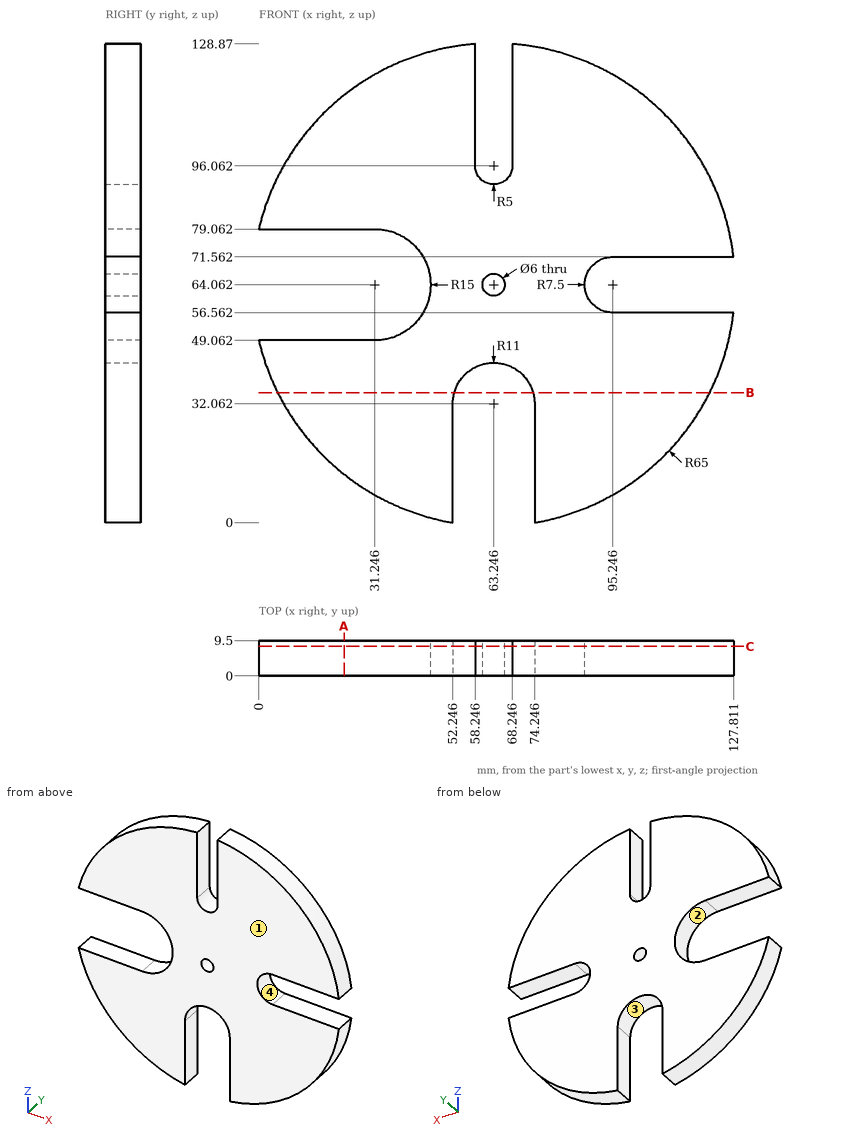
Could you check a few things on this drawing? It's one solid part, dimensions in mm from its lowest x, y, z. Coordinates: 2 decimals unless noted, no trailing zeros. Order: outer loops, then holes, each group sorted by start corner. A loop starts at its lowest first (then second) coordinate and runs counter-clockwise, first axis right, second up. Notation, with made-up numbers: M -28,1 L 7,1 A23 cw 7,12 Z; hole C -37,-34.5 d11. An arc over 180 degrees is marked long. Use one line per item in the form item = value. Start each with the question number.
1. Please list where these lines run through material, in increasing order: line 1 (X direction, y = 2.5, z = 96) (1 decimal); line 2 (Z direction, x = 39.5, y = 8.5) (1 decimal); line 3 (Z direction, x = 15, y = 5.25) (1 decimal).
2. Suppose I cut it at C-C on y = 8. Write out the boundary of the cut face in (x, z) (1 decimal).
3. Suppose I cut it at B-B on z = 35. Write out the boundary of the cut face in (x, y) (1 decimal), then the cut area to 3 significant figures.
4. Suppose I cut it at A-A on x = 23. Write out the boundary of the cut face in (y, z) (1 decimal).
5. We'd pull the mould along X, two halves only. Please class the marked faces 1, 2, 3 and 4: +X half, -X half, draft (parallel to the pull), parting line (faces both ways), or undercut.
6. For pin 1 (1.5 mm diameter, centred on x = 79, y = 1, fed in from -Z); pin 2 (5 mm diameter, centred on y = 4, z = 19.5, fed in from +X); pin 3 (5 mm diameter, centred on x = 114, y = 5.5, fed in from -Z) (1 decimal); pin 4 (1.5 mm diameter, centred on x = 26, z = 115.5, fed in from -Y), each with a flat end and sliding along its axis, tell me the tip position at first contact or that it passes through.
Geometry says:
q1.line_1 = 6.6 to 58.2, 68.2 to 119.9
q1.line_2 = 3.6 to 51.5, 76.6 to 124.6
q1.line_3 = 20.5 to 49.1, 79.1 to 107.6
q2.outline = M 0,49.1 A65 ccw 52.2,0 L 52.2,32.1 A11 cw 74.2,32.1 L 74.2,0 A65 ccw 127.8,56.6 L 95.2,56.6 A7.5 cw 95.2,71.6 L 127.8,71.6 A65 ccw 68.2,128.9 L 68.2,96.1 A5 cw 58.2,96.1 L 58.2,128.9 A65 ccw 0,79.1 L 31.2,79.1 A15 cw 31.2,49.1 Z; hole C 63.2,64.1 d6
q3.outline = M 5.1,0 L 52.6,0 L 52.6,9.5 L 5.1,9.5 Z; M 73.8,0 L 121.4,0 L 121.4,9.5 L 73.8,9.5 Z
q3.area = 903 mm^2
q4.outline = M 0,13 L 9.5,13 L 9.5,49.1 L 0,49.1 Z; M 0,79.1 L 9.5,79.1 L 9.5,115.1 L 0,115.1 Z
q5.face_1 = draft
q5.face_2 = -X half
q5.face_3 = undercut
q5.face_4 = +X half
q6.pin_1 = 0.82
q6.pin_2 = 112.8
q6.pin_3 = 20.5
q6.pin_4 = 0
